For this review, take the finished solid that the model builds, in its own axes (mm). A direction names the side the tool comes from. Give positions to 0.01 mm unless a question says otherwise; leave off trailing zeros. Order: outer loops, then holes, each group sorted by start corner. A loop starts at its lowest first (then second) coordinate and runs counter-clockwise, first axis right, second up.
Item 1: Consider section D-D (z = 7.25). Give the boundary of the cut face in (x, y).
Item 2: The part is to be moulded in two halves that separate along Z. For faces 1 (the cylindrical face through (-0.69, -2.58, -3.1)), 2 (the flat face through (3, 0, -3)), 3 (the cylindrical face through (-2.75, -0.63, -12.4)), say which applies: released by +Z, released by -Z, zero draft, split by the parting line, or undercut.
Item 3: Consider section B-B (x = 0). Give the boundary of the cut face in (y, z) (3 decimals).
Item 4: For P1, Ø4, axis at x = 9, z = -10, coming from the -Y side; P2, Ø1.5, axis at x = -5.5, y = -2.5, coming from the +Z side, all flat-tipped, find the tip position at first contact; note any pin that passes through.
Item 5: For probe 1 along Y at (x, z) = (-7.5, 10); probe 2 along X at (y, z) = (-2.35, -2.25); probe 3 along Z at (x, y) = (2, -2.4), list the stretches that pass through material, from the lowest coordinate up.
Item 6: Consider section C-C (y = -4.65). Give the boundary of the cut face in (x, z) (3 decimals), plus the area to 3 significant figures.
Item 7: Consider section A-A (z = 0). Give the boundary of the cut face in (x, y) (3 decimals), plus the area to 3 significant figures.
Item 8: Machinability: for faces 4 (the cylindrical face through (-2.75, -4.44, -12.4)), 5 (the flat face through (3, -3.81, -8)), which of the approach directions +Z, -Z, +X, -X, +Y, -Y give a long, thin tool a straight path to every point of the face, cutting with its end or side? Answer none if there is none.
```python
from build123d import *

# Parameters (mm, degrees)
F0_R     = 12.7
F1_DEPTH = 1.27
F2_R     = 8.255
F3_DEPTH = 2.54
F4_R     = 12.7
F5_DEPTH = 1.27
F6_R     = 3.175
F7_DEPTH = 25.4


with BuildPart() as f1:
    # F0 (on Front) → F1 (new body)
    with BuildSketch(Plane.XZ):
        Circle(F0_R)
    extrude(amount=F1_DEPTH)

    # F2 (on face) → F3 (join)
    with BuildSketch(Plane.XZ.offset(1.27)):
        Circle(F2_R)
    extrude(amount=F3_DEPTH)

    # F4 (on face) → F5 (join)
    with BuildSketch(Plane.XZ.offset(3.81)):
        Circle(F4_R)
    extrude(amount=F5_DEPTH)

    # F6 (on face) → F7 (cut)
    with BuildSketch(Plane.XZ.offset(5.08)):
        Circle(F6_R)
    extrude(amount=-F7_DEPTH, mode=Mode.SUBTRACT)


solid = f1.part
```
Resolved:
1. outline: (-10.43, -5.08) - (10.43, -5.08) - (10.43, -3.81) - (3.95, -3.81) - (3.95, -1.27) - (10.43, -1.27) - (10.43, 0) - (-10.43, 0) - (-10.43, -1.27) - (-3.95, -1.27) - (-3.95, -3.81) - (-10.43, -3.81) - close
2. face 1: undercut
2. face 2: zero draft
2. face 3: split by the parting line
3. outline: (-5.08, -12.7) - (-3.81, -12.7) - (-3.81, -8.255) - (-1.27, -8.255) - (-1.27, -12.7) - (0, -12.7) - (0, -3.175) - (-5.08, -3.175) - close; (-5.08, 3.175) - (0, 3.175) - (0, 12.7) - (-1.27, 12.7) - (-1.27, 8.255) - (-3.81, 8.255) - (-3.81, 12.7) - (-5.08, 12.7) - close
4. P1: stops at y = -5.08
4. P2: stops at z = 6.75
5. probe 1: y = -5.08 to -3.81, -1.27 to 0
5. probe 2: x = -7.94 to -2.24, 2.24 to 7.94
5. probe 3: z = -8.01 to -2.47, 2.47 to 8.01
6. outline: circle Ø25.4 at (0, 0); hole circle Ø6.35 at (0, 0)
6. area: 475 mm2
7. outline: (-12.7, -5.08) - (-3.175, -5.08) - (-3.175, 0) - (-12.7, 0) - (-12.7, -1.27) - (-8.255, -1.27) - (-8.255, -3.81) - (-12.7, -3.81) - close; (3.175, -5.08) - (12.7, -5.08) - (12.7, -3.81) - (8.255, -3.81) - (8.255, -1.27) - (12.7, -1.27) - (12.7, 0) - (3.175, 0) - close
7. area: 74.2 mm2
8. face 4: +Y, -Y
8. face 5: none
